Study the drawing (mm; zero at the part's minimum x, y, z) and answer. A direction names the side the tool comes from. Coordinates: 2 decimals unless noted, no trailing zeros. Order: outer loops, then holes, each group sorted by start corner. A loop starts at its lowest first (then second) coordinate and runs counter-clockwise, first axis right, second up.
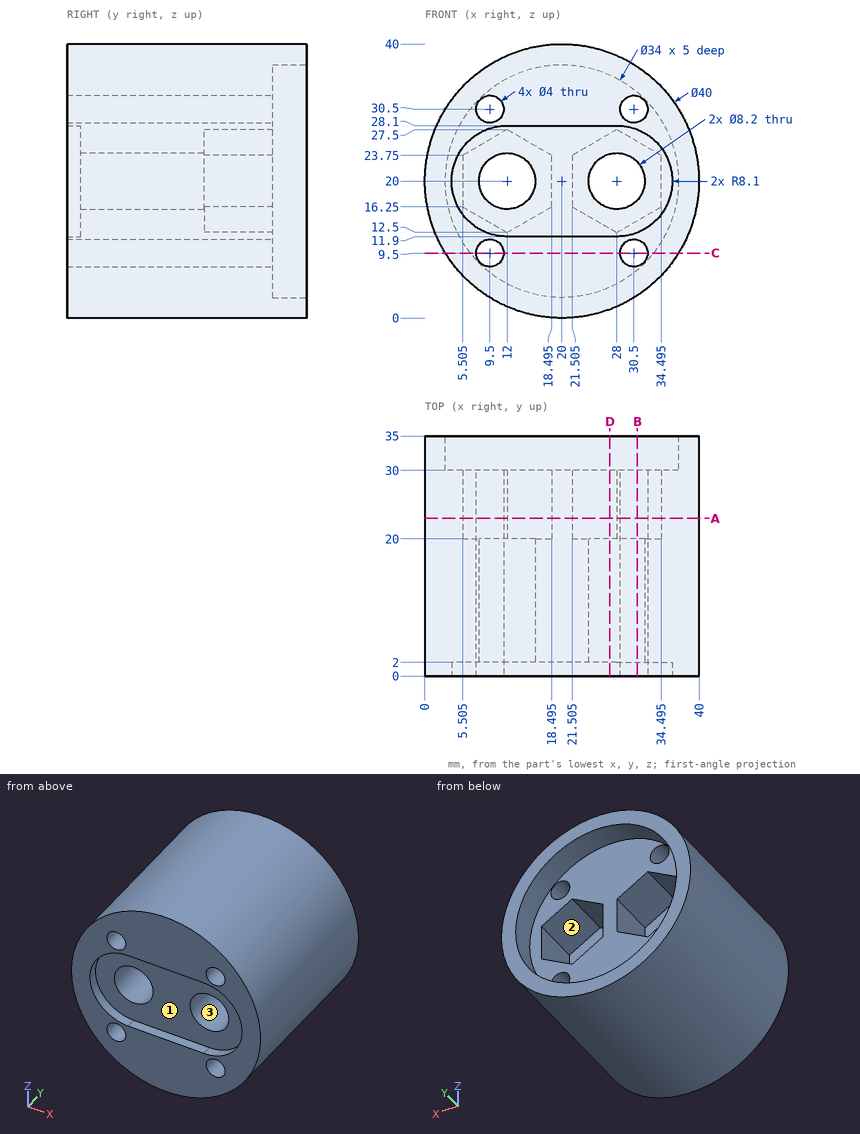
1) A cutting plane is placed at D-D, the plane x = 27. Determine the outline of the cut face in (y, z) (1 decimal).
A:
outline: (0, 1.3) - (35, 1.3) - (35, 4.5) - (30, 4.5) - (30, 13.1) - (20, 13.1) - (20, 16) - (2, 16) - (2, 11.9) - (0, 11.9) - close; (0, 28.1) - (2, 28.1) - (2, 24) - (20, 24) - (20, 26.9) - (30, 26.9) - (30, 35.5) - (35, 35.5) - (35, 38.7) - (0, 38.7) - close
2) A cutting plane is placed at C-C, the plane z = 9.5. Determine the outline of the cut face in (x, y).
A:
outline: (2.98, 0) - (7.5, 0) - (7.5, 30) - (6.63, 30) - (6.63, 35) - (2.98, 35) - close; (11.5, 0) - (28.5, 0) - (28.5, 30) - (11.5, 30) - close; (32.5, 0) - (37.02, 0) - (37.02, 35) - (33.37, 35) - (33.37, 30) - (32.5, 30) - close
3) Flat-ended cylindrical pins translate along their axes: pin 1 Ø10 at (y, z) = (24, 26.5) entering from +X; pin 2 Ø4.5 at (x, z) = (9.5, 30.5) entering from +Y; pin 3 Ø1 at (x, y) = (28.5, 19) entering from +Z; pin 4 Ø8 at (x, z) = (30.5, 18) entering from +Y. Find the tip coordinate at first contact, or state that the pin passes through.
A:
pin 1: stops at x = 39.94
pin 2: stops at y = 35
pin 3: stops at z = 38.33
pin 4: stops at y = 30
4) A cutting plane is placed at B-B, the plane x = 31. Determine the outline of the cut face in (y, z) (1 decimal).
A:
outline: (0, 3.3) - (35, 3.3) - (35, 7) - (30, 7) - (30, 7.6) - (0, 7.6) - close; (0, 11.4) - (30, 11.4) - (30, 14.2) - (20, 14.2) - (20, 17.2) - (2, 17.2) - (2, 12.5) - (0, 12.5) - close; (0, 27.5) - (2, 27.5) - (2, 22.8) - (20, 22.8) - (20, 25.8) - (30, 25.8) - (30, 28.6) - (0, 28.6) - close; (0, 32.4) - (30, 32.4) - (30, 33) - (35, 33) - (35, 36.7) - (0, 36.7) - close
5) Which of the six approach directions +Z, -Z, +X, -X, +Y, -Y give full straight-line access (tool end or side, diameter ignored) to the marked faces 1, 2 and 3?
A:
face 1: -Y
face 2: +Y
face 3: +Y, -Y
6) Straight lines are drawn through the part: line 1 (X direction, y = 13.75, z = 20); line 2 (Z direction, x = 20, y = 32); line 3 (Z direction, x = 30.5, y = 8.5). For each, find the intervals that lie inside material, in ascending order.
A:
line 1: x = 0 to 7.9, 16.1 to 23.9, 32.1 to 40
line 2: z = 0 to 3, 37 to 40
line 3: z = 2.98 to 7.5, 11.5 to 16.75, 23.25 to 28.5, 32.5 to 37.02
7) A cutting plane is placed at A-A, the plane y = 23. State how many separate pieces and enclosed holes the cut face has, and give its area (3 significant figures).
A:
separate pieces: 1
enclosed holes: 6
area: 914 mm2
